Source: CAD feature listing. Evaluate the final solid. Frame: model axes, mm. A direction names the side the tool comes from. Give positions to 0.01 mm unless a question says otherwise; leave off trailing zeros. Write each loop counter-clockwise with the first axis right and the second up, starting at its lowest first coordinate (ties: lowest second). Pieces come first, ordered by that corner, then holes. Notation, with made-up numbers: (-38, -8) -> (-10, -8) arc R24 cw to (-10, 20) -> close; hole circle Ø1 at (-32.5, 8.5). An arc over 180 degrees is marked (long way). Write item = value, one per line.
from build123d import *

# Parameters (mm, degrees)
CROQUIS1_W                 = 20
CROQUIS1_H                 = 35
CROQUIS1_R                 = 5
SALIENTE_EXTRUIR1_DEPTH    = 20
CROQUIS2_R                 = 2
SALIENTE_EXTRUIR2_DEPTH    = 8
CORTAR_EXTRUIR1_DEPTH      = 131.371097716
CORTAR_EXTRUIR1_DEPTH_BACK = 131.371097716
CROQUIS3_R                 = 5.5
CROQUIS4_W                 = 11
CROQUIS4_H                 = 11
CORTAR_EXTRUIR2_DEPTH      = 18
CROQUIS7_W                 = 16
CROQUIS7_H                 = 13.5
CORTAR_EXTRUIR3_DEPTH      = 1.5


with BuildPart() as part:
    # Croquis1 → Saliente-Extruir1 (new body)
    with BuildSketch(Plane(origin=(0, 0, 0), x_dir=(1, 0, 0), z_dir=(0, 1, 0))):
        with Locations((63.781004701, -82.04140038)):
            Rectangle(CROQUIS1_W, CROQUIS1_H)
        with Locations(Location((63.781004701, -89.54140038, 0), (0, 0, 270))):
            Circle(CROQUIS1_R, mode=Mode.SUBTRACT)
        with Locations(Location((63.781004701, -74.54140038, 0), (0, 0, 270))):
            Circle(CROQUIS1_R, mode=Mode.SUBTRACT)
    extrude(amount=SALIENTE_EXTRUIR1_DEPTH)

    # Croquis2 → Saliente-Extruir2 (add)
    with BuildSketch(Plane(origin=(73.781004701, 0, 0), x_dir=(0, 0, -1), z_dir=(1, 0, 0))):
        with Locations(Location((-74.54140038, 12.2, 0), (0, 0, 180))):
            Circle(CROQUIS2_R)
    extrude(amount=SALIENTE_EXTRUIR2_DEPTH)

    # Croquis3 → Cortar-Extruir1 (cut, two sides: drawn at the far end of the back side and taken through both)
    with BuildSketch(Plane(origin=(0, 20, 0), x_dir=(1, 0, 0), z_dir=(0, 1, 0)).offset(-CORTAR_EXTRUIR1_DEPTH_BACK)):
        with Locations(Location((63.781004701, -74.54140038, 0), (0, 0, 270))):
            Circle(CROQUIS3_R)
        with Locations(Location((63.781004701, -89.54140038, 0), (0, 0, 270))):
            Circle(CROQUIS3_R)
    extrude(amount=CORTAR_EXTRUIR1_DEPTH + CORTAR_EXTRUIR1_DEPTH_BACK, mode=Mode.SUBTRACT)

    # Croquis4 → Cortar-Extruir2 (cut)
    with BuildSketch(Plane(origin=(81.781004701, 0, 0), x_dir=(0, 0, -1), z_dir=(1, 0, 0))):
        with Locations((-74.54140038, 12.2)):
            Rectangle(CROQUIS4_W, CROQUIS4_H)
    extrude(amount=-CORTAR_EXTRUIR2_DEPTH, mode=Mode.SUBTRACT)

    # Croquis7 → Cortar-Extruir3 (cut)
    with BuildSketch(Plane(origin=(73.781004701, 0, 0), x_dir=(0, 0, -1), z_dir=(1, 0, 0))):
        with Locations((-74.54140038, 10.95)):
            Rectangle(CROQUIS7_W, CROQUIS7_H)
    extrude(amount=-CORTAR_EXTRUIR3_DEPTH, mode=Mode.SUBTRACT)


solid = part.part
(1) Pull-direction query (Z, two-part tool) for faces 1 (the face through (53.781, 10, 82)), 2 (the face through (64, 10, 99.541)), 3 (the face through (73, 11, 82.541)); classes: pulls with the +Z half, pulls with the -Z half, needs draft (parallel to the pull), parting line crosses it, or undercut.
Values follow:
face_1 = needs draft
face_2 = pulls with the +Z half
face_3 = undercut
(2) First-contact query: pin 1 (6 mm diameter, centred on x = 64.5, z = 76.5, fed in from +Y); pin 2 (4 mm diameter, centred on y = 13.5, z = 76.5, fed in from +X); pin 3 (5 mm diameter, centred on y = 13, z = 79, fed in from +X). Flat tips, straight axial feed; report the tip coordinate or a pass-through.
Values follow:
pin_1 = through
pin_2 = 59.96
pin_3 = 72.28
(3) Section query D-D (z = 68). Return loops of the section in (x, y), plus the area to 3 significant figures.
Values follow:
outline = (53.78, 0) -> (73.78, 0) -> (73.78, 4.2) -> (72.28, 4.2) -> (72.28, 17.7) -> (73.78, 17.7) -> (73.78, 20) -> (53.78, 20) -> close
area = 380 mm2
(4) Section query A-A (z = 79). Return loops of the section in (x, y), plus the area to 3 significant figures.
Values follow:
outline = (53.78, 0) -> (60.56, 0) -> (60.56, 20) -> (53.78, 20) -> close; (67, 0) -> (73.78, 0) -> (73.78, 4.2) -> (72.28, 4.2) -> (72.28, 6.7) -> (67, 6.7) -> close; (67, 17.7) -> (73.78, 17.7) -> (73.78, 20) -> (67, 20) -> close
area = 193 mm2
(5) Section query B-B (x = 65.5). Return loops of the section in (y, z), plus the area to 3 significant figures.
Values follow:
outline = (0, 64.54) -> (20, 64.54) -> (20, 69.32) -> (17.7, 69.32) -> (17.7, 69.04) -> (6.7, 69.04) -> (6.7, 69.32) -> (0, 69.32) -> close; (0, 79.77) -> (6.7, 79.77) -> (6.7, 80.04) -> (17.7, 80.04) -> (17.7, 79.77) -> (20, 79.77) -> (20, 84.32) -> (0, 84.32) -> close; (0, 94.77) -> (20, 94.77) -> (20, 99.54) -> (0, 99.54) -> close
area = 276 mm2
(6) Section query C-C (y = 15.25). Return loops of the section in (x, z), plus the area to 3 significant figures.
Values follow:
outline = (53.78, 64.54) -> (73.78, 64.54) -> (73.78, 66.54) -> (72.28, 66.54) -> (72.28, 69.04) -> (63.78, 69.04) arc R5.5 cw to (63.78, 80.04) -> (72.28, 80.04) -> (72.28, 82.54) -> (73.78, 82.54) -> (73.78, 99.54) -> (53.78, 99.54) -> close; hole circle Ø11 at (63.78, 89.54)
area = 440 mm2
(7) Material intervals for line 1 (Z direction, x = 63.5, y = 16.25); line 2 (Y direction, x = 69, z = 77.5); line 3 (Z direction, x = 63.25, y = 7.75), sorted ascending.
Values follow:
line_1 = 64.54 to 69.05, 80.03 to 84.05, 95.03 to 99.54
line_2 = 0 to 6.7, 17.7 to 20
line_3 = 64.54 to 69.07, 80.02 to 84.07, 95.02 to 99.54
(8) Access query for faces 4 (the face through (73.781, 10, 86)), 5 (the face through (70, 6.7, 75)). Directions: +Z, -Z, +X, -X, +Y, -Y. A direction counts if a zero-diameter tool reaches every point of the face in a straight line with its end or side. Return the directions, or none.
Values follow:
face_4 = +Z, -Z, +X, +Y, -Y
face_5 = +X
